Here's the drawing with two shaded views (mm, measured from the low corner). I have some questions. A direction names the side the tool comes from. Give positions to 0.01 mm unless a question says otherwise; leave off trailing zeros. Loops run counter-clockwise (first coordinate to the right, second up) from the corner with the lowest first, then second, coordinate; pieces in that order, holes last. Notation, with made-up numbers: M -26.75,-3 L -7.75,-3 A19 ccw -7.75,19 Z; hole C -39.5,-1.75 d11. An arc over 180 degrees is marked long. Put each result on its own line as item: value. Start each with the question number.
1) Imagine slicing it at A-A (y = 8). Write out the boundary of the cut face in (x, z), then the cut area to 3 significant figures.
2) For the marked faces 1 and 2, which set-ups out of +Z, -Z, +X, -X, +Y, -Y let a thin tool reach every point of the face, with its end or its side?
3) Imagine slicing it at C-C (z = 4.1). Write out the boundary of the cut face in (x, y).
4) If we mould it in two halves opening along X, with no side actions, what happens to the marked faces 3, 4 and 5? For each: +X half, -X half, draft (parallel to the pull), parting line (faces both ways), or undercut.
5) Imagine slicing it at D-D (x = 14). Write out the boundary of the cut face in (y, z).
6) Please list where these lines run through material, in increasing order: line 1 along Y through (x, z) = (8, 0.4); line 2 along Y through (x, z) = (8, 2.75). Write a range as from..to.
7) For P1, Ø1, axis at y = 2.5, z = 1.5, coming from the -X side (3 decimals); P2, Ø2, axis at x = 13, y = 3, coming from the -Z side; P3, Ø4, axis at x = 7.5, y = 10.5, coming from the -Z side; P4, Ø2, axis at x = 9.5, z = 4, coming from the -Y side, each with a flat end and sliding along its axis, tell me the tip position at first contact or that it passes through.
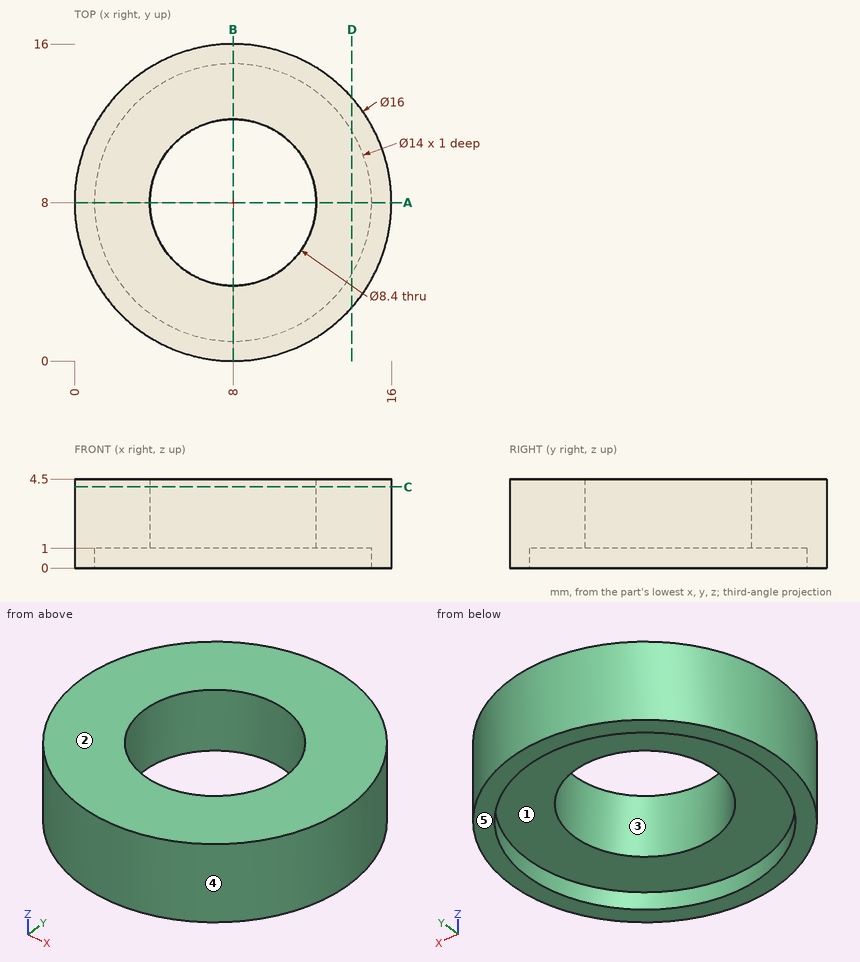
Recorded:
1. outline: M 0,0 L 1,0 L 1,1 L 3.8,1 L 3.8,4.5 L 0,4.5 Z; M 12.2,1 L 15,1 L 15,0 L 16,0 L 16,4.5 L 12.2,4.5 Z
1. area: 28.6 mm²
2. face 1: -Z
2. face 2: +Z, +X, -X, +Y, -Y
3. outline: C 8,8 d16; hole C 8,8 d8.4
4. face 3: undercut
4. face 4: parting line
4. face 5: draft
5. outline: M 2.71,0 L 4.39,0 L 4.39,1 L 11.61,1 L 11.61,0 L 13.29,0 L 13.29,4.5 L 2.71,4.5 Z
6. line 1: 0..1, 15..16
6. line 2: 0..3.8, 12.2..16
7. P1: x = 1.755
7. P2: z = 0
7. P3: z = 1
7. P4: y = 0.02
